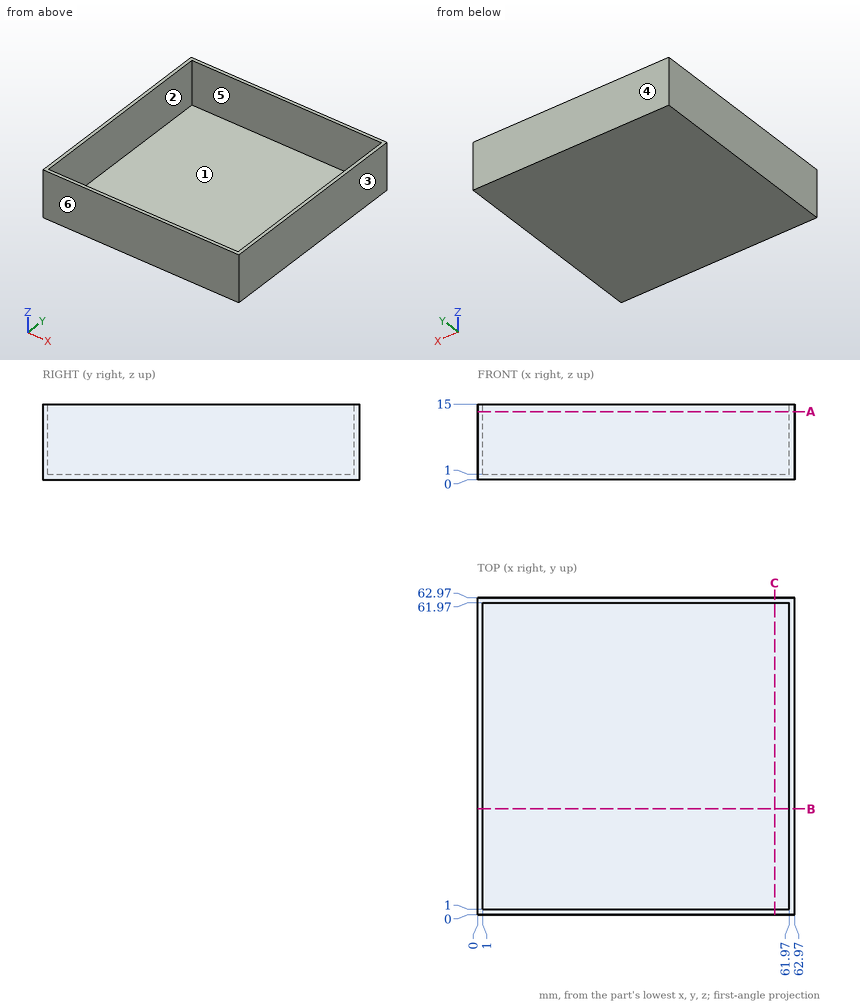
Here's the drawing with two shaded views (mm, measured from the low corner). I have some questions. A direction names the side the tool comes from. Coordinates: 2 decimals unless noted, no trailing zeros. Loops run counter-clockwise (first coordinate to the right, second up) from the corner with the lowest first, then second, coordinate; pieces in that order, holes last. Notation, with made-up numbers: (83.25, 74) -> (121.25, 74) arc R19 ccw to (121.25, 97) -> close; hole circle Ø4 at (37.5, 68.5). An arc over 180 degrees is marked (long way). Answer in a Markdown table with one row per item.
(1) Thinking about a two-plate mould opening in X: for the marked faces 1, 2, 3 and 4, which applies, released by +X, released by -X, zero draft, split by the parting line, or undercut?
Results found:
| item | result |
|---|---|
| face 1 | undercut |
| face 2 | undercut |
| face 3 | released by +X |
| face 4 | zero draft |
(2) If I drill on probe 1 along X at (y, z) = (22.5, 3); probe 2 along Z at (x, y) = (18, 41), over which ranges is the centre line in solid material (lowest first)?
Results found:
| item | result |
|---|---|
| probe 1 | x = 0 to 1, 61.97 to 62.97 |
| probe 2 | z = 0 to 1 |
(3) Will this pin go through, and if not, where does the flat tip stop? pin 1 Ø2 at (x, y) = (11.5, 14.5) entering from +Z.
Results found:
| item | result |
|---|---|
| pin 1 | stops at z = 1 |
(4) For the marked faces 5 and 6, which set-ups out of +Z, -Z, +X, -X, +Y, -Y let a thin tool reach every point of the face, with its end or its side?
Results found:
| item | result |
|---|---|
| face 5 | +Z |
| face 6 | +Z, -Z, +X, -X, -Y |
(5) Imagine slicing it at A-A (z = 13.5). List the corners of the cut face in (x, y) for me.
Results found:
| item | result |
|---|---|
| outline | (0, 0) -> (62.97, 0) -> (62.97, 62.97) -> (0, 62.97) -> close; hole (1, 1) -> (61.97, 1) -> (61.97, 61.97) -> (1, 61.97) -> close |
(6) Imagine slicing it at B-B (y = 21). List the corners of the cut face in (x, z) for me.
Results found:
| item | result |
|---|---|
| outline | (0, 0) -> (62.97, 0) -> (62.97, 15) -> (61.97, 15) -> (61.97, 1) -> (1, 1) -> (1, 15) -> (0, 15) -> close |
